Here's how the part is built. I have some questions about the finished solid (model axes, mm). A direction names the side the tool comes from. Coordinates: 2 decimals unless noted, no trailing zeros. Use a Markdown table: item, result.
```python
from build123d import *

# Parameters (mm, degrees)
PAD_DEPTH       = 5
SKETCH001_R     = 1.52
POCKET_DEPTH    = 0.5
SKETCH002_W     = 1.54
SKETCH002_H     = 9
POCKET001_DEPTH = 0.5
POCKET002_DEPTH = 0.5


with BuildPart() as part:
    # Sketch → Pad (new body)
    with BuildSketch(Plane.YZ):
        Polygon((0, 0), (-30, 0), (-30, 89.600318), (30, 89.600318), (30, 0), align=None)
    extrude(amount=-PAD_DEPTH)

    # Sketch001 → Pocket (cut)
    with BuildSketch(Plane.YZ):
        with Locations((20, 47.266852)):
            Circle(SKETCH001_R)
    extrude(amount=-POCKET_DEPTH, mode=Mode.SUBTRACT)

    # Sketch002 → Pocket001 (cut)
    with BuildSketch(Plane.YZ):
        with Locations((-20, 77.266852)):
            Rectangle(SKETCH002_W, SKETCH002_H)
    extrude(amount=-POCKET001_DEPTH, mode=Mode.SUBTRACT)

    # Sketch003 → Pocket002 (cut)
    with BuildSketch(Plane.YZ):
        with BuildLine():
            ThreePointArc((-15.5, 8.833466), (-15.690919, 8.754384), (-15.77, 8.563466))
            Line((-15.77, 6.103466), (-15.77, 8.563466))
            ThreePointArc((-15.77, 6.103466), (-15.690919, 5.912547), (-15.5, 5.833466))
            Line((-14.5, 5.833466), (-15.5, 5.833466))
            ThreePointArc((-14.5, 5.833466), (-14.309081, 5.912547), (-14.23, 6.103466))
            Line((-14.23, 8.563466), (-14.23, 6.103466))
            ThreePointArc((-14.23, 8.563466), (-14.309081, 8.754384), (-14.5, 8.833466))
            Line((-15.5, 8.833466), (-14.5, 8.833466))
        make_face()
    extrude(amount=-POCKET002_DEPTH, mode=Mode.SUBTRACT)


solid = part.part
```
1. I need wall thicknesses on probe 1 along Z at (x, y) = (-0.3, 20). Which ranges of the line are inside material? Lowest first, please.
Answers follow:
| item | result |
|---|---|
| probe 1 | z = 0 to 45.75, 48.79 to 89.6 |
2. Will these pins go through, and if not, where does the flat tip stop? pin 1 Ø2.5 at (y, z) = (20.5, 47) entering from +X; pin 2 Ø0.5 at (y, z) = (-20, 78) entering from +X.
Answers follow:
| item | result |
|---|---|
| pin 1 | stops at x = 0 |
| pin 2 | stops at x = -0.5 |
3. We'd pull the mould along Y, two halves only. Please class faces 3 (the face through (-0.246, 18.88, 48.294)), 4 (the face through (-2, -30, 44)), 5 (the face through (0, 0, 45)): +Y half, -Y half, draft (parallel to the pull), parting line (faces both ways), or undercut.
Answers follow:
| item | result |
|---|---|
| face 3 | undercut |
| face 4 | -Y half |
| face 5 | draft |
4. Which directions (+Z, -Z, +X, -X, +Y, -Y) give clear straight access to the entire face, cutting with the end or side of a thin tool? Please do faces 1 (the face through (-0.5, 20, 47)), 2 (the face through (-5, 0, 45)).
Answers follow:
| item | result |
|---|---|
| face 1 | +X |
| face 2 | +Z, -Z, -X, +Y, -Y |
